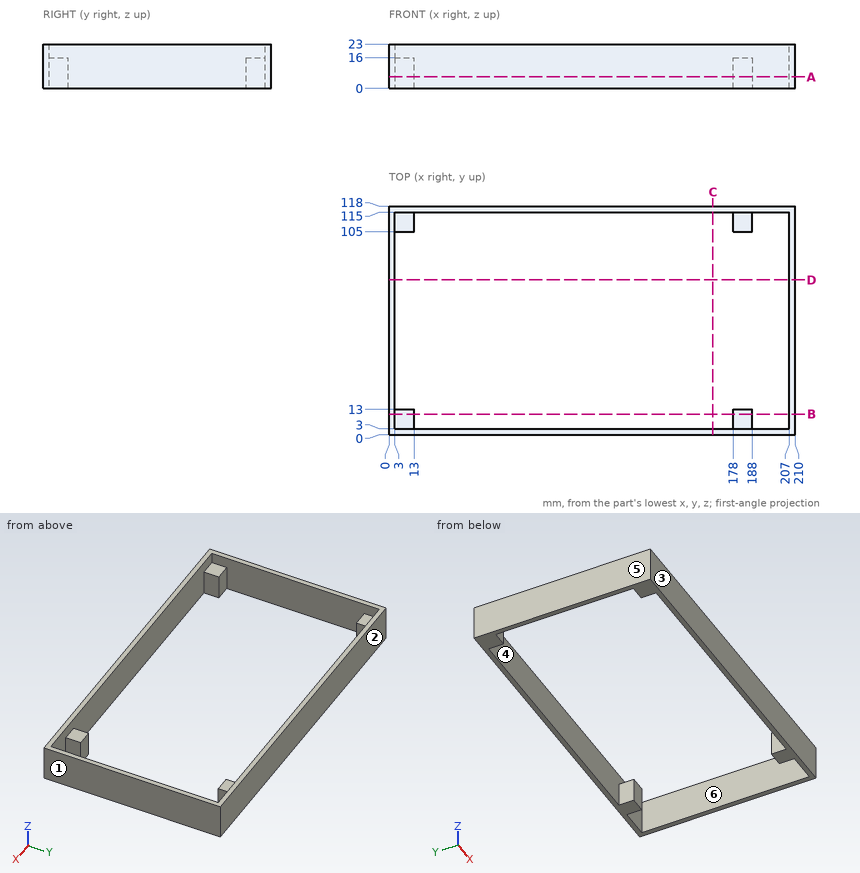
Geometry check sheet. Reference: drawing and pictorial views, mm from the part's lowest x, y, z. A direction names the side the tool comes from. Coordinates: 2 decimals unless noted, no trailing zeros. Write each loop counter-clockwise with the first axis right and the second up, starting at its lowest first coordinate (ties: lowest second). Pieces come first, ordered by that corner, then holes. Notation, with made-up numbers: M 60.5,87 L 72.5,87 A23 cw 72.5,117 Z; hole C -25,-31.75 d11. An arc over 180 degrees is marked long. Use one line per item in the form item = value.
Item 1: Sectioned sample at B-B, the plane y = 10.5. Record the cut outline in (x, z), and give its area (3 significant figures).
Answer below:
outline = M 0,0 L 13,0 L 13,16 L 3,16 L 3,23 L 0,23 Z; M 178,0 L 188,0 L 188,16 L 178,16 Z; M 207,0 L 210,0 L 210,23 L 207,23 Z
area = 458 mm^2
Item 2: Release check for a two-part mould opening along Y. For the marked faces 1, 2, 3 and 4 record: pulls with the +Y half, pulls with the -Y half, needs draft (parallel to the pull), parting line crosses it, or undercut.
Answer below:
face_1 = needs draft
face_2 = pulls with the +Y half
face_3 = pulls with the -Y half
face_4 = undercut
Item 3: Sectioned sample at D-D, the plane y = 80. Record the cut outline in (x, z).
Answer below:
outline = M 0,0 L 3,0 L 3,23 L 0,23 Z; M 207,0 L 210,0 L 210,23 L 207,23 Z
Item 4: Gauge pin test, flat end, axial feed: pin 1 Ø5 at (x, y) = (183, 112) entering from +Z. Record the tip position at first contact, or that the pin passes through.
Answer below:
pin_1 = 16
Item 5: Sectioned sample at C-C, the plane x = 167.5. Record the cut outline in (y, z), and give its area (3 significant figures).
Answer below:
outline = M 0,0 L 3,0 L 3,23 L 0,23 Z; M 115,0 L 118,0 L 118,23 L 115,23 Z
area = 138 mm^2
Item 6: Sectioned sample at A-A, the plane z = 6. Record the cut outline in (x, y), and give its area (3 significant figures).
Answer below:
outline = M 0,0 L 210,0 L 210,118 L 0,118 Z; hole M 3,13 L 13,13 L 13,3 L 178,3 L 178,13 L 188,13 L 188,3 L 207,3 L 207,115 L 188,115 L 188,105 L 178,105 L 178,115 L 13,115 L 13,105 L 3,105 Z
area = 2,330 mm^2
Item 7: Set-up check for the marked faces 5 and 6: record each of +Z, -Z, +X, -X, +Y, -Y from which the full face is reachable in a straight line by a thin tool's end or side.
Answer below:
face_5 = +Z, -Z, -X, +Y, -Y
face_6 = +Z, -Z
Item 8: Material ranges on L1, parallel to X at y = 101, z = 19.25; L2, parallel to Y at x = 190, z = 5.25; L3, parallel to Y at x = 178.5, z = 13, recorded low to high. Write a range as from..to.
Answer below:
L1 = 0..3, 207..210
L2 = 0..3, 115..118
L3 = 0..13, 105..118
